Geometry: final body of the model. Coordinates: model frame, mm. A direction names the side the tool comes from. Give positions to 0.01 mm unless a question says otherwise; leave off trailing zeros. Order: outer loops, then holes, each group sorted by start corner. A loop starts at its lowest first (then second) coordinate and runs counter-clockwise, first axis right, second up. Notation, with made-up numbers: (-10.75, 29) - (18.25, 29) arc R8 ccw to (18.25, 41) - close; hole circle Ø2 at (17, 30). An arc over 180 degrees is marked (long way). Put each result on its own line as item: value. Start each with the question number.
1. Section C-C on z = 14. Return the cut outline in (x, y), plus the area to 3 significant figures.
2. Ray query, line 1 along Y through (x, z) = (-5, 5.5); line 2 along Z through (x, y) = (11.5, 17.5); line 3 along X through (y, z) = (-7, 1). Return the intervals inside material, ascending. Write a range as from..to.
3. Set-up query: faces 1 (the flat face through (0, -15.5, 12)), 2 (the flat face through (10.5, 0, 12)), 3 (the flat face through (-7.384, -3, -9)), 4 (the flat face through (0, 11.519, -7)), 5 (the flat face through (0, -11.519, -10)). Return all of +Z, -Z, +X, -X, +Y, -Y with unobstructed straight access to the full face (end or side cutting, diameter ignored); none if empty.
4. First-contact query: P1, Ø3, axis at x = -2.5, z = 6.5, coming from the -Y side; P2, Ø3, axis at x = -1, z = -12, coming from the -Y side; P3, Ø3, axis at y = -0.5, z = -10, coming from the -X side. Flat tips, straight axial feed; report the tip coordinate or a pass-through.
5. Section D-D on y = 4. Return the cut outline in (x, z).
6. Section A-A on y = -14. Return the cut outline in (x, z).
7. Section B-B on x = -4.25. Return the cut outline in (y, z), plus the area to 3 significant figures.
from build123d import *

# Parameters (mm, degrees)
SKETCH1_W           = 21
SKETCH1_H           = 31
BOSS_EXTRUDE1_DEPTH = 25
SKETCH2_W           = 28
SKETCH2_H           = 38
BOSS_EXTRUDE2_DEPTH = 5
SKETCH3_W           = 14.768534612
SKETCH3_H           = 23.038215668
BOSS_EXTRUDE3_DEPTH = 10
CHAMFER1_SIZE       = 5
CHAMFER1_SIZE2      = 20


with BuildPart() as part:
    # Sketch1 → Boss-Extrude1 (new body)
    with BuildSketch(Plane.XY):
        Rectangle(SKETCH1_W, SKETCH1_H)
    extrude(amount=BOSS_EXTRUDE1_DEPTH)

    # Sketch2 → Boss-Extrude2 (add)
    with BuildSketch(Plane(origin=(0, 0, 0), x_dir=(-1, 0, 0), z_dir=(0, 0, -1))):
        Rectangle(SKETCH2_W, SKETCH2_H)
    extrude(amount=BOSS_EXTRUDE2_DEPTH)

    # Sketch3 → Boss-Extrude3 (add)
    with BuildSketch(Plane(origin=(0, 0, -5), x_dir=(-1, 0, 0), z_dir=(0, 0, -1))):
        Rectangle(SKETCH3_W, SKETCH3_H)
    extrude(amount=BOSS_EXTRUDE3_DEPTH)

    # Chamfer1
    chamfer1_edges = [part.edges().sort_by_distance(p)[0] for p in [
        (0, 11.519107834, -15),
    ]]
    chamfer1_side = [part.faces().sort_by_distance(p)[0] for p in [
        (0, 11.519107834, -10),
    ]]
    chamfer(chamfer1_edges, length=CHAMFER1_SIZE, length2=CHAMFER1_SIZE2, reference=chamfer1_side[0])


solid = part.part
Resolved:
1. outline: (-10.5, -15.5) - (10.5, -15.5) - (10.5, 15.5) - (-10.5, 15.5) - close
1. area: 651 mm^2
2. line 1: -15.5..15.5
2. line 2: -5..0
2. line 3: -10.5..10.5
3. face 1: +Z, +X, -X, -Y
3. face 2: +Z, +X, +Y, -Y
3. face 3: -Z, -X, +Y, -Y
3. face 4: -Z, +X, -X, +Y
3. face 5: -Z, +X, -X, -Y
4. P1: y = -15.5
4. P2: y = -11.52
4. P3: x = -7.38
5. outline: (-14, -5) - (-7.38, -5) - (-7.38, -11.88) - (7.38, -11.88) - (7.38, -5) - (14, -5) - (14, 0) - (10.5, 0) - (10.5, 25) - (-10.5, 25) - (-10.5, 0) - (-14, 0) - close
6. outline: (-14, -5) - (14, -5) - (14, 0) - (10.5, 0) - (10.5, 25) - (-10.5, 25) - (-10.5, 0) - (-14, 0) - close
7. outline: (-19, -5) - (-11.52, -5) - (-11.52, -15) - (-8.48, -15) - (11.52, -10) - (11.52, -5) - (19, -5) - (19, 0) - (15.5, 0) - (15.5, 25) - (-15.5, 25) - (-15.5, 0) - (-19, 0) - close
7. area: 1,150 mm^2
